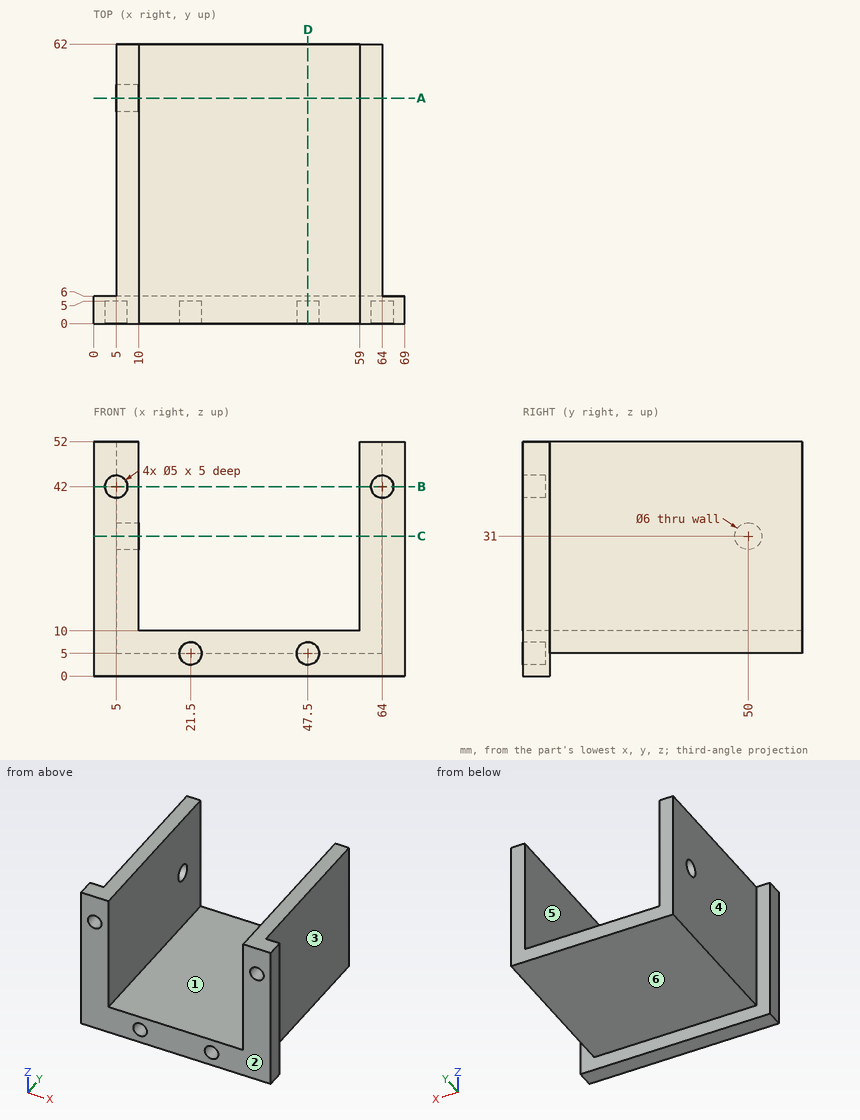
Source: three-view drawing plus pictorial views. Frame: mm from the lowest corner of the part. A direction names the side the tool comes from. Round coordinates to 2 decimals unless told otherwise and drop trailing zeros. Write each loop counter-clockwise with the first axis right and the second up, starting at its lowest first coordinate (ties: lowest second). Pieces come first, ordered by that corner, then holes. Notation, with made-up numbers: M -31.5,89.5 L -1.5,89.5 A17 ccw -1.5,109.5 Z; hole C 81,76.5 d11. An arc over 180 degrees is marked long. Use CSV: the item, a comma, the result in double quotes. Start each with the question number.
Q1. First-contact query: P1, Ø3, axis at x = 47.5, z = 5, coming from the -Y side; P2, Ø21, axis at y = 36, z = 40, coming from the +X side; P3, Ø7, axis at y = 50, z = 31, coming from the -X side; P4, Ø5.5, axis at x = 4.5, z = 43, coming from the -Y side. Flat tips, straight axial feed; report the tip coordinate or a pass-through.
Q2. Cut plane C-C on z = 31. Output: boundary loops of the cut face in (x, y), plus the area to 3 significant figures.
Q3. Line query: line 1 (X direction, y = 3.35, z = 5); line 2 (X direction, y = 2, z = 42); line 3 (Z direction, x = 21.5, y = 3.8). Output: solid intervals per line, ascending. Write a range as from..to.
Q4. Cut plane B-B on z = 42. Output: boundary loops of the cut face in (x, y).
Q5. Cut plane D-D on x = 47.5. Output: boundary loops of the cut face in (y, z), plus the area to 3 significant figures.
Q6. Cut plane A-A on y = 50. Output: boundary loops of the cut face in (x, z).
Q7. Access query for the marked faces 4, 5 and 6. Directions: +Z, -Z, +X, -X, +Y, -Y. A direction counts if a zero-diameter tool reaches every point of the face in a straight line with its end or side. Return the directions, or none.
Q8. Pull-direction query (X, two-part tool) for the marked faces 1, 2 and 3; classes: +X half, -X half, draft (parallel to the pull), parting line (faces both ways), or undercut.
Results found:
1,P1,"y = 5"
1,P2,"x = 64"
1,P3,"x = 5"
1,P4,"y = 0"
2,outline,"M 0,0 L 10,0 L 10,47 L 5,47 L 5,6 L 0,6 Z; M 5,53 L 10,53 L 10,62 L 5,62 Z; M 59,0 L 69,0 L 69,6 L 64,6 L 64,62 L 59,62 Z"
2,area,"650 mm^2"
3,line 1,"0..19, 24..45, 50..69"
3,line 2,"0..2.5, 7.5..10, 59..61.5, 66.5..69"
3,line 3,"0..2.5, 7.5..10"
4,outline,"M 0,0 L 2.5,0 L 2.5,5 L 7.5,5 L 7.5,0 L 10,0 L 10,62 L 5,62 L 5,6 L 0,6 Z; M 59,0 L 61.5,0 L 61.5,5 L 66.5,5 L 66.5,0 L 69,0 L 69,6 L 64,6 L 64,62 L 59,62 Z"
5,outline,"M 0,0 L 6,0 L 6,5 L 62,5 L 62,10 L 0,10 L 0,7.5 L 5,7.5 L 5,2.5 L 0,2.5 Z"
5,area,"315 mm^2"
6,outline,"M 5,5 L 64,5 L 64,52 L 59,52 L 59,10 L 10,10 L 10,28 L 5,28 Z; M 5,34 L 10,34 L 10,52 L 5,52 Z"
7,face 4,"+Z, -Z, -X, +Y"
7,face 5,"+Z, +Y, -Y"
7,face 6,"-Z, +X, -X, +Y"
8,face 1,"undercut"
8,face 2,"draft"
8,face 3,"+X half"
